```python
from build123d import *

# Parameters (mm, degrees)
SKETCH1_W           = 14
SKETCH1_H           = 20
BOSS_EXTRUDE1_DEPTH = 13.98
SKETCH2_R           = 0.825
CUT_EXTRUDE1_DEPTH  = 23.168455066
SKETCH6_W           = 14
SKETCH6_H           = 20
CUT_EXTRUDE2_DEPTH  = 1.5
SKETCH7_R           = 4.55
BOSS_EXTRUDE2_DEPTH = 1.5


with BuildPart() as part:
    # Sketch1 → Boss-Extrude1 (new body)
    with BuildSketch(Plane(origin=(0, 0, 0), x_dir=(1, 0, 0), z_dir=(0, 1, 0))):
        Rectangle(SKETCH1_W, SKETCH1_H)
    extrude(amount=BOSS_EXTRUDE1_DEPTH)

    # Sketch2 → Cut-Extrude1 (cut, through all)
    with BuildSketch(Plane(origin=(7, 0, 0), x_dir=(0, 0, -1), z_dir=(1, 0, 0))):
        with Locations((8, 5.62)):
            Circle(SKETCH2_R)
        with Locations((-8, 5.62)):
            Circle(SKETCH2_R)
    extrude(amount=-CUT_EXTRUDE1_DEPTH, mode=Mode.SUBTRACT)

    # Sketch6 → Cut-Extrude2 (cut)
    with BuildSketch(Plane.XZ):
        Rectangle(SKETCH6_W, SKETCH6_H)
    extrude(amount=-CUT_EXTRUDE2_DEPTH, mode=Mode.SUBTRACT)

    # Sketch7 → Boss-Extrude2 (add)
    with BuildSketch(Plane.XZ.offset(-1.5)):
        with Locations(Location((0, 0, 0), (0, 0, 270))):
            Circle(SKETCH7_R)
    extrude(amount=BOSS_EXTRUDE2_DEPTH)


solid = part.part
```
Geometry check sheet. Reference: the model listing, model coordinates, mm. A direction names the side the tool comes from. Coordinates: 2 decimals unless noted, no trailing zeros. Write each loop counter-clockwise with the first axis right and the second up, starting at its lowest first coordinate (ties: lowest second). Pieces come first, ordered by that corner, then holes. Notation, with made-up numbers: M 21.25,36 L 30.25,36 A32 cw 30.25,71 Z; hole C 77.25,-22 d8. An arc over 180 degrees is marked long. One line per item, written item: value. Start each with the question number.
(1) Scan lines: line 1 along Z through (x, y) = (2.75, 5.5); line 2 along Y through (x, z) = (-0.5, -8) (3 decimals); line 3 along Z through (x, y) = (-2.5, 5). Record each from-to range of solid material in increasing order. Write a range as [from, to].
(2) Sectioned sample at D-D, the plane z = 0. Enter the section's corners in (x, y).
(3) Tool access check on faces 1 (the face through (0, 8, -10)), 2 (the face through (-2.77, 0.76, 3.61)). Record the directions out of +Z, -Z, +X, -X, +Y, -Y that give a thin tool (end or side, any length) a straight path to the whole face; none if there is none.
(4) Sectioned sample at B-B, the plane z = -8. Enter the section's corners in (x, y) (3 decimals).
(5) Release check for a two-part mould opening along Y. For faces 3 (the face through (0.1, 5.3, 7.24)), 4 (the face through (0.098, 5.868, -8.787)), 5 (the face through (0, 1.5, 5)), 6 (the face through (0, 8, 10)) record: released by +Y, released by -Y, zero draft, split by the parting line, or undercut.
(6) Sectioned sample at A-A, the plane y = 5.62. Enter the section's corners in (x, z) (3 decimals), and give its area (3 significant figures).
(7) Sectioned sample at C-C, the plane x = 0. Enter the section's corners in (y, z) (3 decimals).
Filled sheet:
1. line 1: [-10, -8.82], [-7.18, 7.18], [8.82, 10]
1. line 2: [1.5, 4.795], [6.445, 13.98]
1. line 3: [-10, -8.54], [-7.46, 7.46], [8.54, 10]
2. outline: M -7,1.5 L -4.55,1.5 L -4.55,0 L 4.55,0 L 4.55,1.5 L 7,1.5 L 7,13.98 L -7,13.98 Z
3. face 1: -Z, +X, -X, +Y, -Y
3. face 2: -Y
4. outline: M -7,1.5 L 7,1.5 L 7,4.795 L -7,4.795 Z; M -7,6.445 L 7,6.445 L 7,13.98 L -7,13.98 Z
5. face 3: undercut
5. face 4: undercut
5. face 5: released by -Y
5. face 6: zero draft
6. outline: M -7,-10 L 7,-10 L 7,-8.825 L -7,-8.825 Z; M -7,-7.175 L 7,-7.175 L 7,7.175 L -7,7.175 Z; M -7,8.825 L 7,8.825 L 7,10 L -7,10 Z
6. area: 234 mm²
7. outline: M 0,-4.55 L 1.5,-4.55 L 1.5,-10 L 13.98,-10 L 13.98,10 L 1.5,10 L 1.5,4.55 L 0,4.55 Z; hole C 5.62,-8 d1.65; hole C 5.62,8 d1.65
